```python
from build123d import *

# Parameters (mm, degrees)
F0_R     = 1.5
F1_DEPTH = 5


with BuildPart() as f1:
    # F0 (on Top) → F1 (new body)
    with BuildSketch(Plane.XY):
        with BuildLine():
            Line((28.575, 31.67), (-28.575, 31.67))
            ThreePointArc((-28.575, 31.67), (-33.9065851301, 29.4615851301), (-36.115, 24.13))
            Line((-36.115, 24.13), (-36.115, -24.13))
            ThreePointArc((-36.115, -24.13), (-33.9065851301, -29.4615851301), (-28.575, -31.67))
            Line((-28.575, -31.67), (28.575, -31.67))
            ThreePointArc((28.575, -31.67), (33.9065851301, -29.4615851301), (36.115, -24.13))
            Line((36.115, -24.13), (36.115, 24.13))
            ThreePointArc((36.115, 24.13), (33.9065851301, 29.4615851301), (28.575, 31.67))
        make_face()
        with Locations((-28.575, -24.13)):
            Circle(F0_R, mode=Mode.SUBTRACT)
        Polygon((6.2527900536, -11.5708104593), (9.2793256044, -14.0073262155), (-0.9104009134, -27.1782091798), (-11.4204209558, -14.0073262155), (-8.51109229, -11.5708104593), (-5.5128769018, -15.1508381907), (-4.1845976375, -10.3244902566), (2.4567989167, -10.3244902566), (3.3706848119, -15.1508381907), (3.7498176424, -14.6798956216), align=None, mode=Mode.SUBTRACT)
        Polygon((-23.2801141861, -2.1800489627), (-3.2509050798, -27.2801313549), (-19.2656442523, -22.165434435), align=None, mode=Mode.SUBTRACT)
        with Locations((28.575, -24.13)):
            Circle(F0_R, mode=Mode.SUBTRACT)
        Polygon((0.7662613061, -27.2293109447), (20.8395048976, -2.2951872088), (17.5112579018, -22.4489029497), (1.4907777077, -27.2293109447), align=None, mode=Mode.SUBTRACT)
        Polygon((-9.9460659389, -9.1543504968), (-13.361800462, -12.0149729773), (-23.3147393549, 0.4577904218), (-26.6425088048, 27.1988492459), (-19.0398674458, 15.4525628313), (-12.0270624757, 14.7153204307), (-10.9837119319, 7.7022297044), (-18.4164068339, 8.7475319435), (-18.2800174343, 6.4083864975), (-10.5500826612, 5.114952568), (-9.6885105595, 1.9968850538), (-17.3490952176, 2.7163710911), (-17.2258857638, 0.603268214), (-7.4416000808, -0.7727516371), (-2.0714257844, -7.1850237437), (-2.0714257844, -8.754757233), (-4.9091139808, -8.754757233), (-13.0237422309, -5.51773565), align=None, mode=Mode.SUBTRACT)
        with BuildLine():
            add(Edge.make_bspline(
                [(-1.5434205998, 15.9520953894), (-2.1127854677, 15.8652707774), (-3.1954940882, 15.7001644261), (-4.2268327688, 16.8407808297), (-5.4375210158, 17.6281538425), (-9.2633203303, 23.0989462448), (-12.147068046, 27.2226296365)],
                knots=[0, 0, 0, 0, 0.1812052149, 0.3445812332, 0.5059692848, 1, 1, 1, 1], degree=3))
            Line((-1.5434205998, 15.9520953894), (-1.5434205998, 8.9782960713))
            Line((-1.5434205998, 8.9782960713), (-2.7677833568, 8.9782960713))
            Line((-2.7677833568, 8.9782960713), (-1.0155849159, 4.7854543664))
            Line((-1.0155849159, 4.7854543664), (1.2114524143, 8.9782960713))
            Line((1.2114524143, 8.9782960713), (-0.495339511, 8.9782960713))
            Line((-0.495339511, 8.9782960713), (-0.495339511, 15.5966216698))
            add(Edge.make_bspline(
                [(2.392585855, 16.7120974511), (2.1150017163, 16.4235156809), (1.4856865312, 15.7692675998), (0.2149107712, 15.6585198064), (-0.495339511, 15.5966216698)],
                knots=[0, 0, 0, 0, 0.4410892114, 1, 1, 1, 1], degree=3))
            Line((2.392585855, 16.7120974511), (10.12203563, 27.2226296365))
            Line((10.12203563, 27.2226296365), (5.2505019121, 1.9477001624))
            Line((5.2505019121, 1.9477001624), (5.1744488655, 1.8045151419))
            add(Edge.make_bspline(
                [(5.1744488655, 1.8045151419), (4.7180148969, 1.6646463966), (3.4212599775, 1.14619058), (2.2473178638, -0.6256342161), (1.4829438878, -1.7792999279)],
                knots=[0.1136874814, 0.1136874814, 0.1136874814, 0.1136874814, 0.4229066187, 1, 1, 1, 1], degree=3))
            Line((1.4829438878, -1.7792999279), (-3.7846511696, -1.7792999279))
            add(Edge.make_bspline(
                [(-7.5035453774, 2.4273574818), (-6.9701059824, 2.2073427858), (-5.6561009128, 1.6653872637), (-4.4820682586, -0.4955979623), (-3.7846511696, -1.7792999279)],
                knots=[0, 0, 0, 0, 0.4059644878, 1, 1, 1, 1], degree=3))
            Line((-7.5035453774, 2.4273574818), (-12.147068046, 27.2226296365))
        make_face(mode=Mode.SUBTRACT)
        with Locations((-28.575, 24.13)):
            Circle(F0_R, mode=Mode.SUBTRACT)
        Polygon((22.2602374852, 2.7163710911), (11.0789202031, -11.5303234741), (8.1275883001, -9.1543504968), (11.0552490609, -5.51773565), (2.9398098122, -8.754757233), (0, -8.754757233), (0, -7.1850237437), (5.1622066744, -0.7727516371), (15.4377110302, 0.603268214), (16.2226036191, 2.7163710911), (8.1275883001, 2.1730016451), (8.6015986256, 5.0433022481), (16.2226036191, 6.0638510984), (17.1265321758, 8.4974248905), (9.0981954709, 8.029313758), (10.2221901556, 14.8355001374), (17.1265321758, 15.7600787614), (26.3624843102, 27.2325830574), align=None, mode=Mode.SUBTRACT)
        with Locations((28.575, 24.13)):
            Circle(F0_R, mode=Mode.SUBTRACT)
    extrude(amount=F1_DEPTH)


solid = f1.part
```
Can you work these out from the model? Positions are in its coordinate system, mm. A direction names the side the tool comes from. Coordinates: 2 decimals unless noted, no trailing zeros. Write item = value, one per line. Start each with the question number.
Q1. On a 3-axis mill with a long thin cutter (end or side, diameter ignored), from which of +Z, -Z, +X, -X, +Y, -Y can I reach the whole of each face in a straight line? I mean faces 5 (the face through (-0.495, 12, 2)), 6 (the face through (0, 31.67, 2)). Say none if no direction works.
Q2. If we section it at A-A, the plane z = 3.25: State how many separate pieces and enclosed holes the cut face has, then the cut area to 3 significant figures.
Q3. If I drill on L1, parallel to X at y = -22, z = 2.6 (3 decimals); L2, parallel to X at y = 22, z = 2 (3 decimals); L3, parallel to Y at x = -29.5, z = 4.7, over which ranges is the centre line in solid material (lowest first)? Write a range as [from, to].
Q4. I'm going to push a flat-ended pin straight in: pin 1 (1.8 mm diameter, centred on x = 28.575, y = -24.13, fed in from +Z). Where does the tip first touch, or does it pass through?
Q5. Thinking about a two-plate mould opening in X: for faces 1 (the face through (-36.115, 0, 2)), 2 (the face through (-9.99, -12.81, 2.46)), 3 (the face through (13.63, 15.29, 2.46)), 4 (the face through (0, -31.67, 2)), which applies, released by +X, released by -X, zero draft, split by the parting line, or undercut?
Check sheet entries:
q1.face_5 = +Z, -Z
q1.face_6 = +Z, -Z, +X, -X, +Y
q2.separate_pieces = 1
q2.enclosed_holes = 10
q2.area = 3,040 mm²
q3.L1 = [-36.115, -19.299], [-7.464, -5.042], [3.096, 4.976], [17.585, 36.115]
q3.L2 = [-36.115, -25.996], [-23.278, -11.169], [-8.469, 6.281], [9.115, 22.15], [25.487, 36.115]
q3.L3 = [-31.61, -25.31], [-22.95, 22.95], [25.31, 31.61]
q4.pin_1 = through
q5.face_1 = released by -X
q5.face_2 = undercut
q5.face_3 = undercut
q5.face_4 = zero draft
